```python
from build123d import *

# Parameters (mm, degrees)
EXTRUDE_1_DEPTH           = 5
HOLE_WIZARD_1_D           = 5.5
HOLE_WIZARD_1_CBORE_D     = 10
HOLE_WIZARD_1_CBORE_DEPTH = 5.7
CHAMFER_1_SIZE            = 2
SKETCH_5_R                = 1
CUT_EXTRUDE_1_DEPTH       = 44.588989435


with BuildPart() as part:
    # 草图1 → 凸台-拉伸1 (new, symmetric)
    with BuildSketch(Plane.XY):
        Polygon((0, 0), (0, 30), (12, 30), (12, 12), (30, 12), (30, 0), align=None)
    extrude(amount=EXTRUDE_1_DEPTH, both=True)

    # 打孔尺寸(%根据)内六角圆柱头螺钉的类型1 (through all)
    with Locations(Plane.XY.offset(5)):
        with Locations((6, 22), (22, 6)):
            CounterBoreHole(HOLE_WIZARD_1_D / 2, HOLE_WIZARD_1_CBORE_D / 2, HOLE_WIZARD_1_CBORE_DEPTH)

    # 倒角1
    chamfer_1_edges = [part.edges().sort_by_distance(p)[0] for p in [
        (0, 0, 0),
        (0, 30, 0),
        (12, 30, 0),
        (30, 12, 0),
        (30, 0, 0),
    ]]
    chamfer(chamfer_1_edges, length=CHAMFER_1_SIZE)

    # 草图5 → 切除-拉伸1 (cut, through all)
    with BuildSketch(Plane.XY.offset(5)):
        with Locations((12, 12)):
            Circle(SKETCH_5_R)
    extrude(amount=-CUT_EXTRUDE_1_DEPTH, mode=Mode.SUBTRACT)


solid = part.part
```
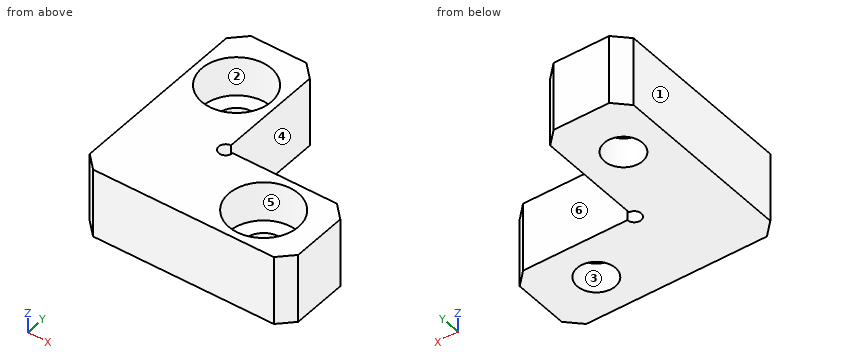
Geometry check sheet. Reference: the model listing, model coordinates, mm. Face numbers are marked on the shaded views. A direction names the side the tool comes from. Coordinates: 2 decimals unless noted, no trailing zeros. Write each loop counter-clockwise with the first axis right and the second up, starting at its lowest first coordinate (ties: lowest second). Pieces come first, ordered by that corner, then holes. Notation, with made-up numbers: M 86.25,52 L 97.25,52 A24 cw 97.25,66 Z; hole C 31,80 d3. An arc over 180 degrees is marked long. Use one line per item in the form item = value. Start each with the question number.
1) Section check D-D on x = 18. Enter the section's corners in (y, z), and give its area (3 significant figures).
2) Section check B-B on x = 22. Enter the section's corners in (y, z), and give its area (4 significant figures).
3) Section check A-A on y = 6. Enter the section's corners in (x, z), and give its area (3 significant figures).
4) Release check for a two-part mould opening along Y. For the marked faces 3, 4, 5 and 6 record: pulls with the +Y half, pulls with the -Y half, needs draft (parallel to the pull), parting line crosses it, or undercut.
5) Go/stop test with flat-tipped pins: pin 1 Ø1.6 at (x, y) = (12, 12) entering from +Z; pin 2 Ø4 at (x, z) = (16, -2) entering from +Y. Record where each tip stops, or that it passes through.
6) Set-up check for the marked faces 1 and 2: record each of +Z, -Z, +X, -X, +Y, -Y from which the full face is reachable in a straight line by a thin tool's end or side.
7) Thickness scan on probe 1 along Y at (x, z) = (22, -3.15); probe 2 along Y at (x, z) = (6, -3.4); probe 3 along X at (y, z) = (5.75, 3). Record the ranges inside material, lowest first. Write a range as from..to.
8) Section check C-C on z = -2.5. Enter the section's corners in (x, y).
Responses:
q1.outline = M 0,-5 L 12,-5 L 12,5 L 9,5 L 9,-0.7 L 3,-0.7 L 3,5 L 0,5 Z
q1.area = 85.8 mm2
q2.outline = M 0,-5 L 3.25,-5 L 3.25,-0.7 L 1,-0.7 L 1,5 L 0,5 Z; M 8.75,-5 L 12,-5 L 12,5 L 11,5 L 11,-0.7 L 8.75,-0.7 Z
q2.area = 39.35 mm2
q3.outline = M 0,-5 L 19.25,-5 L 19.25,-0.7 L 17,-0.7 L 17,5 L 0,5 Z; M 24.75,-5 L 30,-5 L 30,5 L 27,5 L 27,-0.7 L 24.75,-0.7 Z
q3.area = 219 mm2
q4.face_3 = undercut
q4.face_4 = needs draft
q4.face_5 = undercut
q4.face_6 = pulls with the +Y half
q5.pin_1 = through
q5.pin_2 = 12
q6.face_1 = +Z, -Z, -X, +Y, -Y
q6.face_2 = +Z
q7.probe_1 = 0..3.25, 8.75..12
q7.probe_2 = 0..19.25, 24.75..30
q7.probe_3 = 0..17.01, 26.99..30
q8.outline = M 0,2 L 2,0 L 28,0 L 30,2 L 30,10 L 28,12 L 13,12 A1 cw long 12,13 L 12,28 L 10,30 L 2,30 L 0,28 Z; hole C 6,22 d5.5; hole C 22,6 d5.5
